Part model, mm, in its own coordinate system. A direction names the side the tool comes from. Round coordinates to 2 decimals unless told otherwise and drop trailing zeros. Write each loop counter-clockwise with the first axis right and the second up, starting at its lowest first coordinate (ties: lowest second). Pieces come first, ordered by that corner, then holes. Notation, with made-up numbers: (63.25, 43) -> (113.25, 43) arc R15 cw to (113.25, 59) -> close; hole circle Ø7 at (42, -32). An arc over 180 degrees is marked (long way). Return JSON: item names as keys, results as strings. Group by question number.
(1) Drill centre lines: L1, parallel to Y at x = 1.4, z = -6.75; L2, parallel to X at y = 0.15, z = 8.75. Where is each one in solid material? Low to high. Write a range as from..to.
(2) Saw through at A-A (z = -0.75). List the corners of the cut face in (x, y).
(3) Tool access for faces 1 (the flat face through (-2, 0.992, 0)), 2 (the flat face through (2, -0.992, 0)), 3 (the flat face through (-0.992, -2, 0)): list every direction of +Z, -Z, +X, -X, +Y, -Y with a clear straight run to the whole face (end or side of a thin tool).
(4) Drop flat-ended pins along their axis: pin 1 Ø0.5 at (y, z) = (-1.5, -3) entering from -X; pin 2 Ø1.2 at (y, z) = (1.5, 5) entering from -X; pin 3 Ø1.5 at (x, z) = (1, -3) entering from +Y. Give the stop position or say it passes through.
from build123d import *

# Parameters (mm, degrees)
SKETCH1_R           = 2.38125
EXTRUDE1_DEPTH      = 11.6765625
FILLET1_R           = 1.016
EXTRUDE2_DEPTH      = 13.152481882
EXTRUDE2_DEPTH_BACK = 13.152481882


with BuildPart() as part:
    # Sketch1 → Extrude1 (new, symmetric)
    with BuildSketch(Plane.XY):
        Circle(SKETCH1_R)
    extrude(amount=EXTRUDE1_DEPTH, both=True)

    # Fillet1
    fillet1_edges = [part.edges().sort_by_distance(p)[0] for p in [
        (-2.38125, 0, -11.6765625),
        (-2.38125, 0, 11.6765625),
    ]]
    fillet(fillet1_edges, radius=FILLET1_R)

    # Sketch3 → Extrude2 (cut, two sides: drawn at the far end of the back side and taken through both)
    with BuildSketch(Plane.XY.offset(-EXTRUDE2_DEPTH_BACK)):
        with BuildLine():
            Line((-0.9921875, 2.16469756), (-0.9921875, 1.1191875))
            ThreePointArc((-0.9921875, 1.1191875), (-1.029384939, 1.029384939), (-1.1191875, 0.9921875))
            Line((-1.1191875, 0.9921875), (-2.16469756, 0.9921875))
            ThreePointArc((-2.16469756, 0.9921875), (-1.683798023, 1.683798023), (-0.9921875, 2.16469756))
        make_face()
        with BuildLine():
            Line((-2.16469756, -0.9921875), (-1.1191875, -0.9921875))
            ThreePointArc((-1.1191875, -0.9921875), (-1.029384939, -1.029384939), (-0.9921875, -1.1191875))
            Line((-0.9921875, -1.1191875), (-0.9921875, -2.16469756))
            ThreePointArc((-0.9921875, -2.16469756), (-1.683798023, -1.683798023), (-2.16469756, -0.9921875))
        make_face()
        with BuildLine():
            Line((0.9921875, 2.16469756), (0.9921875, 1.1191875))
            ThreePointArc((0.9921875, 1.1191875), (1.029384939, 1.029384939), (1.1191875, 0.9921875))
            Line((1.1191875, 0.9921875), (2.16469756, 0.9921875))
            ThreePointArc((2.16469756, 0.9921875), (1.683798023, 1.683798023), (0.9921875, 2.16469756))
        make_face()
        with BuildLine():
            Line((0.9921875, -1.1191875), (0.9921875, -2.16469756))
            ThreePointArc((0.9921875, -2.16469756), (1.683798023, -1.683798023), (2.16469756, -0.9921875))
            Line((2.16469756, -0.9921875), (1.1191875, -0.9921875))
            ThreePointArc((1.1191875, -0.9921875), (1.029384939, -1.029384939), (0.9921875, -1.1191875))
        make_face()
    extrude(amount=EXTRUDE2_DEPTH + EXTRUDE2_DEPTH_BACK, mode=Mode.SUBTRACT)


solid = part.part
Computed values:
{
 "1": {"L1": "-0.99..0.99", "L2": "-2.38..2.38"},
 "2": {"outline": "(-2.16, -0.99) -> (-1.12, -0.99) arc R0.13 cw to (-0.99, -1.12) -> (-0.99, -2.16) arc R2.38 ccw to (0.99, -2.16) -> (0.99, -1.12) arc R0.13 cw to (1.12, -0.99) -> (2.16, -0.99) arc R2.38 ccw to (2.16, 0.99) -> (1.12, 0.99) arc R0.13 cw to (0.99, 1.12) -> (0.99, 2.16) arc R2.38 ccw to (-0.99, 2.16) -> (-0.99, 1.12) arc R0.13 cw to (-1.12, 0.99) -> (-2.16, 0.99) arc R2.38 ccw to start"},
 "3": {"face 1": "+Z, -Z, -X, +Y", "face 2": "+Z, -Z, +X, -Y", "face 3": "+Z, -Z, -X, -Y"},
 "4": {"pin 1": "x = -0.99", "pin 2": "x = -2.2", "pin 3": "y = 2.37"}
}
